Can you work these out from the model? Positions are in its coordinate system, mm. Give positions to 0.01 mm unless a question says otherwise; leave off trailing zeros. Write each loop counter-clockwise with the first axis right and the second up, starting at its lowest first coordinate (ties: lowest second). Pieces come first, ordered by that corner, then holes. Notation, with made-up numbers: M 83.5,45.5 L 131.5,45.5 A12 cw 131.5,52.5 Z; hole C -4,53 d6. An arc over 180 degrees is marked long. Answer as CSV lines item,"result". Start each with the question number.
```python
from build123d import *

# Parameters (mm, degrees)
BOSS_EXTRUDE1_DEPTH            = 4.7625
BOSS_EXTRUDE1_DEPTH_BACK       = 4.7625
SKETCH3_W                      = 382.27
SKETCH3_H                      = 31.75
FILLET1_R                      = 0.314325
TAP_DRILL_FOR_10_32_TAP1_D     = 4.0386
TAP_DRILL_FOR_10_32_TAP1_DEPTH = 25.4
TAP_DRILL_FOR_10_32_TAP1_TIP   = 1.213317848
TAP_DRILL_FOR_10_32_TAP2_D     = 4.0386
TAP_DRILL_FOR_10_32_TAP2_DEPTH = 25.4
TAP_DRILL_FOR_10_32_TAP2_TIP   = 1.213317848
CUT_EXTRUDE1_DEPTH             = 194.812621187


with BuildPart() as part:
    # Sketch3 → Boss-Extrude1 (new, two sides: drawn at the far end of the back side and taken through both)
    with BuildSketch(Plane(origin=(0, 0, 0), x_dir=(1, 0, 0), z_dir=(0, 1, 0)).offset(-BOSS_EXTRUDE1_DEPTH_BACK)):
        Rectangle(SKETCH3_W, SKETCH3_H)
    extrude(amount=BOSS_EXTRUDE1_DEPTH + BOSS_EXTRUDE1_DEPTH_BACK)

    # Fillet1
    fillet1_edges = [part.edges().sort_by_distance(p)[0] for p in [
        (0, 4.7625, 15.875),
        (0, -4.7625, -15.875),
        (0, 4.7625, -15.875),
        (0, -4.7625, 15.875),
    ]]
    fillet(fillet1_edges, radius=FILLET1_R)

    # Tap Drill for #10-32 Tap1
    with Locations(Plane.ZY.offset(191.135)):
        with Locations((-11.43, 0), (11.43, 0)):
            Hole(TAP_DRILL_FOR_10_32_TAP1_D / 2, depth=TAP_DRILL_FOR_10_32_TAP1_DEPTH)
            with Locations((0, 0, -(TAP_DRILL_FOR_10_32_TAP1_DEPTH + TAP_DRILL_FOR_10_32_TAP1_TIP / 2))):  # 118° drill point
                Cone(0, TAP_DRILL_FOR_10_32_TAP1_D / 2, TAP_DRILL_FOR_10_32_TAP1_TIP, mode=Mode.SUBTRACT)

    # Tap Drill for #10-32 Tap2
    with Locations(Plane(origin=(191.135, 0, 0), x_dir=(0, 0, -1), z_dir=(1, 0, 0))):
        with Locations((-11.43, 0), (11.43, 0)):
            Hole(TAP_DRILL_FOR_10_32_TAP2_D / 2, depth=TAP_DRILL_FOR_10_32_TAP2_DEPTH)
            with Locations((0, 0, -(TAP_DRILL_FOR_10_32_TAP2_DEPTH + TAP_DRILL_FOR_10_32_TAP2_TIP / 2))):  # 118° drill point
                Cone(0, TAP_DRILL_FOR_10_32_TAP2_D / 2, TAP_DRILL_FOR_10_32_TAP2_TIP, mode=Mode.SUBTRACT)

    # Sketch9 → Cut-Extrude1 (cut, through all)
    with BuildSketch(Plane(origin=(0, 0, -15.875), x_dir=(-1, 0, 0), z_dir=(0, 0, -1))):
        with BuildLine():
            Line((159.385, 4.7625), (159.385, 3.175))
            ThreePointArc((159.385, 3.175), (158.45506403, 0.92993597), (156.21, 0))
            Line((156.21, 0), (-156.21, 0))
            ThreePointArc((-156.21, 0), (-158.45506403, 0.92993597), (-159.385, 3.175))
            Line((-159.385, 3.175), (-159.385, 4.7625))
            Line((-159.385, 4.7625), (159.385, 4.7625))
        make_face()
    extrude(amount=-CUT_EXTRUDE1_DEPTH, mode=Mode.SUBTRACT)


solid = part.part
```
1) I need wall thicknesses on L1, parallel to Z at x = -175.25, y = 0 (3 decimals); L2, parallel to X at y = 4, z = -5.5 (3 decimals); L3, parallel to X at y = 2.25, z = 14 (3 decimals). Which ranges of each line are inside material? Lowest first, please. Write a range as from..to.
2) I'm going to push flat-ended pins straight in: P1, Ø3, axis at x = -132.5, y = 0.5, coming from the +Z side (3 decimals); P2, Ø9.5, axis at x = 46.5, z = -2, coming from the +Y side; P3, Ø1, axis at x = 148.5, y = 1.5, coming from the -Z side; P4, Ø3.5, axis at y = 0, z = 11.43, coming from the +X side. Where does each tip first touch, or does it pass through?
3) Thinking about a two-plate mould opening in X: for faces 1 (the flat face through (-2, 0, 0)), 2 (the flat face through (-175, 4.762, 0)), 3 (the flat face through (-191.135, 0, 0)), which applies, released by +X, released by -X, zero draft, split by the parting line, or undercut?
4) I want a section at B-B, the plane x = 104.5. Please give me the cut outline in (y, z) (1 decimal).
Values found:
1,L1,"z = -15.875..-13.449, -9.411..9.411, 13.449..15.875"
1,L2,"x = -191.135..-159.385, 159.385..191.135"
1,L3,"x = -191.135..-159.247, 159.247..191.135"
2,P1,"stops at z = 15.875"
2,P2,"stops at y = 0"
2,P3,"passes through"
2,P4,"stops at x = 165.57"
3,face 1,"undercut"
3,face 2,"zero draft"
3,face 3,"released by -X"
4,outline,"M -4.8,-15.6 A0.3 ccw -4.4,-15.9 L 0,-15.9 L 0,15.9 L -4.4,15.9 A0.3 ccw -4.8,15.6 Z"
